Study the drawing (mm; zero at the part's minimum x, y, z) and answer. Coordinates: 2 decimals unless noted, no trailing zeros. Write each loop counter-clockwise with the first axis right and the second up, starting at its lowest first coordinate (ties: lowest second). Pieces come first, ordered by that corner, then holes. Notation, with made-up numbers: (-30.5, 49.25) -> (-8.5, 49.25) arc R11 cw to (-8.5, 70.25) -> close; hole circle Ø6 at (-16.75, -34.75). An arc over 180 degrees is marked (long way). Write item = value, one per line. Start each with the question number.
1) Section A-A (y = 1.25) is taken. Determine the outline of the cut face in (x, z), plus the area to 3 significant figures.
2) Find the intervals of material crossed by line 1 along Z through (x, y) = (34.5, 1.3); line 2 along X through (y, z) = (3.95, 61); line 3 along X through (y, z) = (1.55, 19), in increasing order. Write a range as from..to.
3) Section C-C (x = 127) is taken. Determine the outline of the cut face in (y, z) (3 decimals).
4) Section B-B (z = 59) is taken. Determine the outline of the cut face in (x, y).
5) Section D-D (z = 9) is taken. Determine the outline of the cut face in (x, y).
6) A flat-ended cylindrical pin translates along its axis: pin 1 Ø2.5 at (y, z) = (3.5, 59.5) entering from -X. Find the tip coordinate at first contact, or state that the pin passes through.
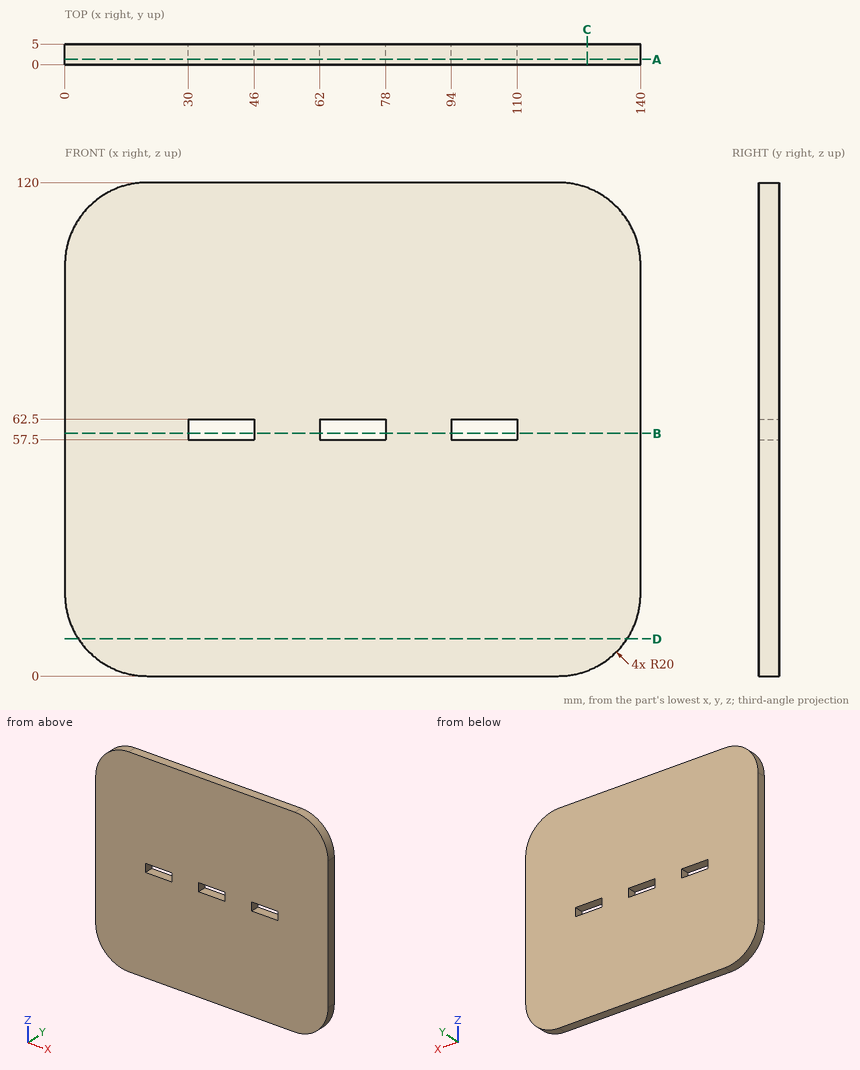
Answer key:
q1.outline = (0, 20) arc R20 ccw to (20, 0) -> (120, 0) arc R20 ccw to (140, 20) -> (140, 100) arc R20 ccw to (120, 120) -> (20, 120) arc R20 ccw to (0, 100) -> close; hole (30, 57.5) -> (46, 57.5) -> (46, 62.5) -> (30, 62.5) -> close; hole (62, 57.5) -> (78, 57.5) -> (78, 62.5) -> (62, 62.5) -> close; hole (94, 57.5) -> (110, 57.5) -> (110, 62.5) -> (94, 62.5) -> close
q1.area = 16,200 mm^2
q2.line_1 = 0..57.5, 62.5..120
q2.line_2 = 0..30, 46..62, 78..94, 110..140
q2.line_3 = 0.03..139.97
q3.outline = (0, 1.265) -> (5, 1.265) -> (5, 118.735) -> (0, 118.735) -> close
q4.outline = (0, 0) -> (30, 0) -> (30, 5) -> (0, 5) -> close; (46, 0) -> (62, 0) -> (62, 5) -> (46, 5) -> close; (78, 0) -> (94, 0) -> (94, 5) -> (78, 5) -> close; (110, 0) -> (140, 0) -> (140, 5) -> (110, 5) -> close
q5.outline = (3.3, 0) -> (136.7, 0) -> (136.7, 5) -> (3.3, 5) -> close
q6.pin_1 = 0
